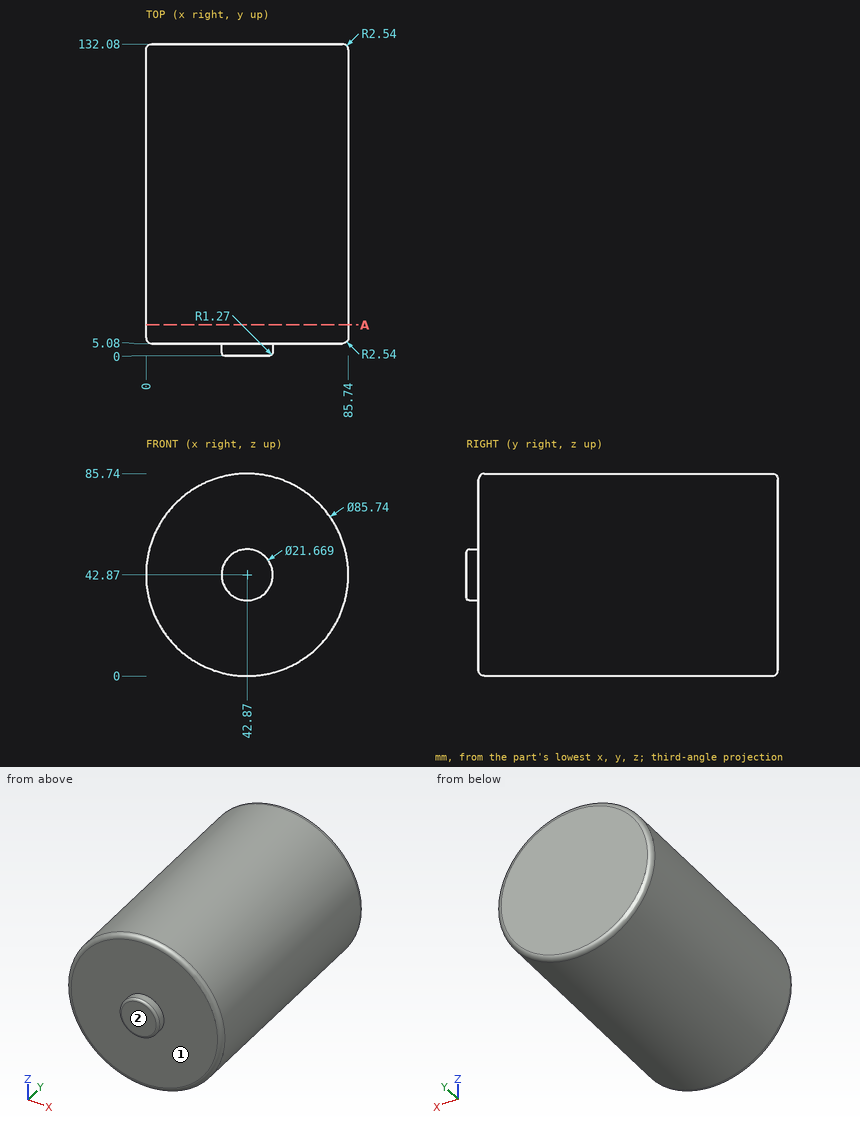
Source: three-view drawing plus pictorial views. Frame: mm from the lowest corner of the part. A direction names the side the tool comes from. Coordinates: 2 decimals unless noted, no trailing zeros. Loops run counter-clockwise (first coordinate to the right, second up) from the corner with the lowest first, then second, coordinate; pieces in that order, holes last. Notation, with made-up numbers: (34, 29) -> (47, 29) arc R22 cw to (47, 47) -> close; hole circle Ø1 at (12.5, 57.5). An arc over 180 degrees is marked (long way). One line per item, written item: value.
(1) Cut plane A-A (y = 13). Output: boundary loops of the cut face in (x, z).
Answer below:
outline: circle Ø85.74 at (42.87, 42.87)
(2) Pin query (flat end, axial travel): pin 1 Ø12 at (x, y) = (46.5, 73.5) entering from +Z; pin 2 Ø10 at (y, z) = (79, 54) entering from -X; pin 3 Ø6 at (y, z) = (37.5, 66) entering from -X. Return the tip coordinate at first contact, or that it passes through.
Answer below:
pin 1: stops at z = 85.74
pin 2: stops at x = 0.44
pin 3: stops at x = 5.02
(3) Ray query, line 1 along Y through (x, z) = (65, 51); line 2 along Z through (x, y) = (41.5, 104); line 3 along X through (y, z) = (18.5, 71). Return the intervals inside material, ascending.
Answer below:
line 1: y = 5.08 to 132.08
line 2: z = 0.02 to 85.72
line 3: x = 10.52 to 75.22
(4) Set-up query: the marked faces 1 and 2. Return all of +Z, -Z, +X, -X, +Y, -Y with unobstructed straight access to the full face (end or side cutting, diameter ignored); none if empty.
Answer below:
face 1: -Y
face 2: +Z, -Z, +X, -X, -Y
